For this review, take the finished solid that the model builds, in its own axes (mm). A direction names the side the tool comes from. Give positions to 0.01 mm unless a question says otherwise; leave off trailing zeros. Order: outer loops, then holes, each group sorted by start corner. A loop starts at its lowest first (then second) coordinate and runs counter-clockwise, first axis right, second up.
Autodesk Inventor part; units mm, degrees
ref_plane "Plano de trabajo1" through (-60, -15, 10) normal (0, 0, 1) x (1, 0, 0)
ref_plane "Plano de trabajo3" through (-60, -13.4, 10) normal (0, 0, 1) x (1, 0, 0)
ref_plane "YZ Plane" through (0, 0, 0) normal (1, 0, 0) x (0, 1, 0)
sketch "Boceto1" plane through (0, 0, 0) normal (0, 0, 1) x (1, 0, 0)
  circle A0 centre (-50, -88) radius 1.5
  circle A1 centre (50, -88) radius 1.5
  circle A2 centre (88, -50) radius 1.5
  circle A3 centre (88, 50) radius 1.5
  circle A4 centre (50, 88) radius 1.5
  circle A5 centre (-50, 88) radius 1.5
  circle A6 centre (-88, 50) radius 1.5
  circle A7 centre (-88, -50) radius 1.5
  arc A8 (29.6244, 31.0386) -> (29.5223, 33.9623) centre (28.2102, 32.4528) ccw
  line L0 (29.6244, 31.0386) -> (9.8759, 11.2901)
  line L1 (-9.8759, 11.2901) -> (-29.6244, 31.0386)
  arc A9 (-29.5223, 33.9623) -> (-29.6244, 31.0386) centre (-28.2102, 32.4528) ccw
  arc A10 (29.5223, 33.9623) -> (-29.5223, 33.9623) centre (0, 0) ccw
  line L2 (100, -100) -> (100, 100)
  line L3 (100, 100) -> (-100, 100)
  line L4 (-100, 100) -> (-100, -100)
  line L5 (-100, -100) -> (100, -100)
  line L6 (10.7339, 9.8854) -> (30.7558, 29.9072)
  arc A11 (30.7558, 29.9072) -> (30.572, 35.1698) centre (28.2102, 32.4528) ccw
  arc A12 (30.572, 35.1698) -> (-30.572, 35.1698) centre (0, 0) ccw
  arc A13 (-30.572, 35.1698) -> (-30.7558, 29.9072) centre (-28.2102, 32.4528) ccw
  line L7 (-30.7558, 29.9072) -> (-12.0679, 11.2194)
  line L8 (31.8102, 5.2085) -> (31.8102, 100)
  line L9 (30.2102, 29.3617) -> (30.2102, 100)
  line L10 (-31.8102, 32.4528) -> (-31.8102, 100)
  line L11 (-30.2102, 31.7383) -> (-30.2102, 100)
  circle A14 centre (55, 0) radius 2.5
  arc A15 (-5.2203, -12.3413) -> (5.2203, -12.3413) centre (0, 0) ccw
  arc A16 (54.4847, -4.9734) -> (5.2203, -12.3413) centre (44.1778, -104.4408) ccw
  arc A17 (54.4847, -4.9734) -> (54.4847, 4.9734) centre (55, 0) ccw
  arc A18 (11.6313, 9.8854) -> (54.4847, 4.9734) centre (44.1778, 104.4408) ccw
  arc A19 (-54.4847, 4.9734) -> (-11.6313, 9.8854) centre (-44.1778, 104.4408) ccw
  arc A20 (-54.4847, 4.9734) -> (-54.4847, -4.9734) centre (-55, 0) ccw
  arc A21 (-5.2203, -12.3413) -> (-54.4847, -4.9734) centre (-44.1778, -104.4408) ccw
  circle A22 centre (0, 0) radius 4
  circle A23 centre (-55, 0) radius 2.5
  arc A24 (9.8759, 11.2901) -> (-9.8759, 11.2901) centre (0, 0) ccw
  line L12 (-30.7558, 29.9072) -> (-10.7339, 9.8854)
  arc A25 (5.2203, 12.3413) -> (-5.2203, 12.3413) centre (0, 0) ccw
  line L13 (10.9657, 10.1171) -> (30.7558, 29.9072)
  arc A26 (30.7558, 29.9072) -> (30.572, 35.1698) centre (28.2102, 32.4528) ccw
  arc A27 (30.572, 35.1698) -> (-30.572, 35.1698) centre (0, 0) ccw
  arc A28 (-30.572, 35.1698) -> (-30.7558, 29.9072) centre (-28.2102, 32.4528) ccw
  line L14 (11.6313, 9.8854) -> (-11.6313, 9.8854)
  line L15 (9.8759, 11.2901) -> (-9.8759, 11.2901)
  point P0 (-30.2102, 32.4528)
  point P1 (30.2102, 32.4528)
  point P2 (31.8102, 32.4528)
  point P3 (-30.2102, 35.4811)
  point P4 (31.8102, 32.4528)
  point P5 (30.2102, 35.4811)
  point P6 (44.1778, 104.4408)
  point P7 (-44.1778, 104.4408)
  dimension "d0" = 1.6
ref_plane "Plano de trabajo1" through (-60, -15, 10) normal (0, 0, 1) x (1, 0, 0)
ref_plane "Plano de trabajo3" through (-60, -13.4, 10) normal (0, 0, 1) x (1, 0, 0)
extrude "Extrusión1" add sketch "Boceto1" along normal up to surface (10 mm away) contours A8 L9 L6 L14 L12 L7 A13 A12 L11 A9 L1 L15 L0 | L9 A12 A11 L6 | L9 L3 L8 A11 A12 | A12 A13 L10 L3 L11
ref_plane "Plano de trabajo5" through (0, 32.4528, 0) normal (-1, 0, 0) x (0, 0, 1)
sketch "Boceto4" plane through (0, 32.4528, 0) normal (-1, 0, 0) x (0, 0, 1)
  line L0 (10, -1.4142) -> (10, -21.1627)
  line L1 (10, 0) -> (10, -1.4142)
  line L2 (10, 67.5472) -> (10, 0)
  line L3 (10, 0) -> (10, 67.5472)
  line L4 (10, -2.5456) -> (10, 0)
  line L5 (10, -22.5674) -> (10, -2.5456)
  line L6 (10, -2.5456) -> (10, -22.5674)
  line L7 (10, 0) -> (10, -2.5456)
  line L8 (10, 67.5472) -> (10, 0)
  line L9 (10, 0) -> (10, 67.5472)
  line L10 (10, -1.4142) -> (10, 0)
  line L11 (10, -21.1627) -> (10, -1.4142)
  line L12 (-103, 70.5472) -> (-78, 70.5472)
  line L13 (-78, 70.5472) -> (-53, 70.5472)
  line L14 (-53, 70.5472) -> (-28, 70.5472)
  line L15 (-28, 70.5472) -> (-3, 70.5472)
  line L16 (-3, 70.5472) -> (22, 70.5472)
  line L17 (22, 70.5472) -> (47, 70.5472)
  line L18 (47, 70.5472) -> (72, 70.5472)
  line L19 (72, 70.5472) -> (97, 70.5472)
  line L20 (97, 70.5472) -> (122, 70.5472)
  line L21 (122, 70.5472) -> (147, 70.5472)
  line L22 (10, -22.5674) -> (63.7597, 70.5472)
  line L23 (10, -22.5674) -> (117.5195, -22.5674) construction
  point P0 (0, -32.4528)
  dimension "d9" = 60
sketch "Boceto5" plane through (-10.7339, 9.8854, 10) normal (0, 0, 1) x (1, 0, 0)
  line L0 (-18.8905, 21.1532) -> (0.858, 1.4047)
  arc A0 (-19.4762, 22.5674) -> (-18.8905, 21.1532) centre (-17.4762, 22.5674) ccw
  line L1 (-19.4762, 90.1146) -> (-19.4762, 22.5674)
  line L2 (-21.0762, 90.1146) -> (-19.4762, 90.1146)
  line L3 (-21.0762, 22.5674) -> (-21.0762, 90.1146)
  arc A1 (-21.0762, 22.5674) -> (-20.0218, 20.0218) centre (-17.4762, 22.5674) ccw
  line L4 (0, 0) -> (-20.0218, 20.0218)
  line L5 (21.4679, 0) -> (0, 0)
  line L6 (41.4897, 20.0218) -> (21.4679, 0)
  arc A2 (41.4897, 20.0218) -> (42.5441, 22.5674) centre (38.9441, 22.5674) ccw
  line L7 (42.5441, 90.1146) -> (42.5441, 22.5674)
  line L8 (40.9441, 90.1146) -> (42.5441, 90.1146)
  line L9 (40.9441, 22.5674) -> (40.9441, 90.1146)
  arc A3 (40.3583, 21.1532) -> (40.9441, 22.5674) centre (38.9441, 22.5674) ccw
  line L10 (20.6098, 1.4047) -> (40.3583, 21.1532)
  line L11 (0.858, 1.4047) -> (20.6098, 1.4047)
  point P0 (10.7339, -9.8854)
sweep "Barrido2" add profiles "Boceto5" path "Boceto4" path curves L22
ref_plane "Plano de trabajo6" through (-31.8102, 100, 0) normal (0, 1, 0) x (1, 0, 0)
split "Dividir2" plane through (-31.8102, 100, 0) removes the side toward (0, 1, 0)
properties part number "Tolva_Salida"
1) Draft analysis for pull direction X (two halves, no side actions). For faces 3 (the face through (-31.81, 82, 21)), 4 (the face through (-0.15, 55.574, 36.378)), 5 (the face through (-30.21, 81, 21)), state which applies: +X half, -X half, draft (parallel to the pull), parting line (faces both ways), or undercut.
Answer sheet:
face 3: -X half
face 4: draft
face 5: undercut
2) Tool access review of faces 1 (the face through (-19.612, 21.026, 4.93)), 2 (the face through (-31.81, 66, 5)): name each direction out of +Z, -Z, +X, -X, +Y, -Y from which nothing blocks a thin tool from reaching the whole face with its end or side.
Answer sheet:
face 1: -Z, +Y
face 2: +Z, -Z, -X, +Y, -Y
3) We need section B-B on z = 7.5. Give the boundary of the cut face in (x, y).
Answer sheet:
outline: (-31.81, 32.45) arc R3.6 ccw to (-30.76, 29.91) - (-12.07, 11.22) - (-10.73, 9.89) - (10.73, 9.89) - (30.76, 29.91) arc R3.6 ccw to (31.81, 32.45) - (31.81, 100) - (30.21, 100) - (30.21, 32.45) arc R2 cw to (29.62, 31.04) - (9.88, 11.29) - (-9.88, 11.29) - (-29.62, 31.04) arc R2 cw to (-30.21, 32.45) - (-30.21, 100) - (-31.81, 100) - close
4) We need section A-A on x = -6.5. Give the boundary of the cut face in (y, z), then the cut area to 3 significant figures.
Answer sheet:
outline: (9.89, 0) - (11.29, 0) - (11.29, 10) - (100, 61.22) - (100, 62.03) - (9.89, 10) - close
area: 86.6 mm2
5) Clearance check with flat-ended pins moving along their axes: pin 1 (5 mm diameter, centred on x = -16.5, z = 23.5, fed in from -Y); pin 2 (6 mm diameter, centred on x = 9, z = 14, fed in from -Y); pin 3 (3 mm diameter, centred on x = 20.5, z = 31.5, fed in from +Y). State where each tip first meets the part, or that it passes through.
Answer sheet:
pin 1: stops at y = 34.03
pin 2: stops at y = 11.62
pin 3: stops at y = 62.15
6) To check wall thickness, follow line 1 (X direction, y = 73.5, z = 3); line 2 (Y direction, x = -4.5, z = 10); line 3 (Y direction, x = -28, z = 42). State the ranges of each line that lie inside material, in increasing order.
Answer sheet:
line 1: x = -31.81 to -30.21, 30.21 to 31.81
line 2: y = 9.89 to 11.29
line 3: y = 82.58 to 84.84
7) We need section D-D on x = 12. Give the boundary of the cut face in (y, z), then the cut area to 3 significant figures.
Answer sheet:
outline: (11.15, 0) - (13.41, 0) - (13.41, 10) - (100, 59.99) - (100, 61.3) - (11.15, 10) - close
area: 137 mm2
